Autodesk Inventor part; units mm, degrees
ref_plane "YZ Plane" through (0, 0, 0) normal (1, 0, 0) x (0, 1, 0)
ref_plane "XZ Plane" through (0, 0, 0) normal (0, 1, 0) x (-1, 0, 0)
ref_plane "XY Plane" through (0, 0, 0) normal (0, 0, 1) x (1, 0, 0)
sketch "Sketch1" plane through (0, 0, 0) normal (0, 1, 0) x (-1, 0, 0)
  line L0 (107.2514, 61.1758) -> (-112.4586, 61.1758)
  line L1 (-112.4586, 61.1758) -> (-112.4586, 42.1258)
  line L2 (-112.4586, 42.1258) -> (107.2514, 42.1258)
  line L3 (107.2514, 42.1258) -> (107.2514, 61.1758)
  point P0 (0, 0)
  dimension "d0" = 219.71
  dimension "d1" = 19.05
extrude "Extrusion1" add sketch "Sketch1" along normal blind 139.7
sketch "Sketch2" plane through (-107.2514, 0, 61.1758) normal (0, 0, 1) x (1, 0, 0)
  line L0 (0, 0) -> (219.71, 0)
  line L1 (0, 139.7) -> (219.71, 139.7)
  line L2 (0, 0) -> (0, 139.7)
  line L3 (219.71, 0) -> (219.71, 139.7)
  point P0 (107.2514, 0)
  point P1 (9.525, 76.2)
  point P2 (9.525, 25.4)
  point P3 (210.185, 25.4)
  point P4 (210.185, 76.2)
  dimension "d4" = 0
  dimension "d5" = 0
  dimension "d6" = 0
  dimension "d7" = 0
  dimension "d8" = 25.4
  dimension "d10" = 9.525
  dimension "d11" = 9.525
  dimension "d57" = 50.8
hole "Hole1" at (-97.7264, 76.2, 61.1758) at (-97.7264, 25.4, 61.1758) at (102.9336, 25.4, 61.1758) at (102.9336, 76.2, 61.1758) direction (0, 0, -1) diameter 6.35 end through all
sketch "Sketch3" plane through (-107.2514, 0, 61.1758) normal (0, 0, 1) x (1, 0, 0)
  line L0 (19.05, 133.35) -> (200.66, 133.35)
  line L1 (200.66, 133.35) -> (200.66, 6.35)
  line L2 (200.66, 6.35) -> (19.05, 6.35)
  line L3 (19.05, 6.35) -> (19.05, 133.35)
  line L4 (0, 0) -> (0, 139.7)
  line L5 (219.71, 0) -> (219.71, 139.7)
  line L6 (219.71, 139.7) -> (0, 139.7)
  line L7 (0, 0) -> (219.71, 0)
  point P0 (107.2514, 0)
  dimension "d19" = 19.05
  dimension "d20" = 19.05
  dimension "d21" = 6.35
  dimension "d22" = 6.35
extrude "Extrusion2" cut sketch "Sketch3" against normal blind 6.35 contours L0 L1 L2 L3
sketch "Sketch6" plane through (0, 139.7, 0) normal (0, 1, 0) x (1, 0, 0)
  line L0 (-88.2014, -54.8258) -> (-107.2514, -54.8258)
  line L1 (-107.2514, -54.8258) -> (-107.2514, -42.1258)
  line L2 (-107.2514, -42.1258) -> (-88.2014, -42.1258)
  line L3 (-88.2014, -42.1258) -> (-88.2014, -54.8258)
  line L4 (112.4586, -42.1258) -> (-107.2514, -42.1258)
  line L5 (-107.2514, -42.1258) -> (-107.2514, -61.1758)
  line L6 (112.4586, -54.8258) -> (93.4086, -54.8258)
  line L7 (93.4086, -54.8258) -> (93.4086, -42.1258)
  line L8 (93.4086, -42.1258) -> (112.4586, -42.1258)
  line L9 (112.4586, -42.1258) -> (112.4586, -54.8258)
  line L10 (112.4586, -61.1758) -> (112.4586, -42.1258)
  line L11 (-107.2514, -61.1758) -> (112.4586, -61.1758)
  point P0 (0, 0)
  dimension "d25" = 0
  dimension "d26" = 12.7
  dimension "d27" = 0
  dimension "d28" = 19.05
  dimension "d32" = 19.05
  dimension "d33" = 0
  dimension "d34" = 6.35
extrude "Extrusion3" cut sketch "Sketch6" against normal blind 254 contours L0 L1 L2 L3 | L4 L9 L6 L7
sketch "Sketch7" plane through (0, 0, 0) normal (0, -1, 0) x (1, 0, 0)
  line L0 (112.4586, 61.1758) -> (112.4586, 42.1258)
  line L1 (112.4586, 42.1258) -> (-107.2514, 42.1258)
  line L2 (-107.2514, 42.1258) -> (-107.2514, 61.1758)
  point P0 (0, 0)
  point P1 (61.6586, 51.6508)
  point P2 (-56.4514, 51.6508)
  point P3 (112.4586, 54.8258)
  point P4 (93.4086, 42.1258)
  point P5 (-88.2014, 42.1258)
  point P6 (-107.2514, 54.8258)
  dimension "d37" = 50.8
  dimension "d38" = 9.525
  dimension "d39" = 50.8
  dimension "d40" = 9.525
hole "Hole2" at (61.6586, 0, 51.6508) at (-56.4514, 0, 51.6508) direction (0, 1, 0) diameter 4.9149 depth 25.4 tip angle 118
sketch "Sketch8" plane through (0, 0, 0) normal (0, -1, 0) x (1, 0, 0)
  line L0 (112.4586, 61.1758) -> (112.4586, 42.1258)
  line L1 (112.4586, 42.1258) -> (-107.2514, 42.1258)
  point P0 (0, 0)
  point P1 (-1.8414, 51.6508)
  point P2 (-1.8414, 51.6508)
  point P3 (112.4586, 54.8258)
  point P4 (93.4086, 42.1258)
  point P5 (-88.2014, 42.1258)
  dimension "d48" = 114.3
  dimension "d49" = 9.525
hole "Hole3" at (-1.8414, 0, 51.6508) direction (0, 1, 0) diameter 4.9149 depth 25.4 tip angle 118
sketch "Sketch9" plane through (-107.2514, 0, 61.1758) normal (0, 0, 1) x (1, 0, 0)
  circle A0 centre (210.185, 76.2) radius 3.175
  line L0 (219.71, 0) -> (219.71, 139.7)
  line L1 (0, 0) -> (0, 139.7)
  point P0 (107.2514, 0)
  point P1 (9.525, 127)
  point P2 (210.185, 127)
  dimension "d58" = 0
  dimension "d59" = 50.8
  dimension "d60" = 9.525
  dimension "d61" = 9.525
hole "Hole4" at (-97.7264, 127, 61.1758) at (102.9336, 127, 61.1758) direction (0, 0, -1) diameter 6.35 depth 25.4 tip angle 118
properties part number "TallFrontWall"
Geometry: final body of the model. Coordinates: model frame, mm. A direction names the side the tool comes from. Round coordinates to 2 decimals unless told otherwise and drop trailing zeros. Order: outer loops, then holes, each group sorted by start corner. A loop starts at its lowest first (then second) coordinate and runs counter-clockwise, first axis right, second up. Notation, with made-up numbers: (67, -1.75) - (95, -1.75) arc R21 cw to (95, 21.25) - close; hole circle Ø3 at (86, -7.5). An arc over 180 degrees is marked (long way). Use CSV: the item, a comma, the result in double quotes. Start each with the question number.
Q1. Material intervals for line 1 along X through (y, z) = (127, 59); line 2 along Y through (x, z) = (57, 58.25); line 3 along X through (y, z) = (102, 59.75), sorted ascending. Write a range as from..to.
Q2. Section query C-C (x = 38). Return loops of the section in (y, z), and give its area (3 significant figures).
Q3. Mould query, pull axis X, two halves, no side actions, for faces 1 (the face through (4, 69, 42.126)), 2 (the face through (4, 6.35, 58)), 3 (the face through (112.459, 69, 58)). Classes: +X half, -X half, draft (parallel to the pull), parting line (faces both ways), or undercut.
Q4. First-contact query: pin 1 (9.5 mm diameter, centred on x = 99.5, y = 39, fed in from -Z); pin 2 (4 mm diameter, centred on y = 109, z = 50, fed in from -X); pin 3 (5 mm diameter, centred on x = 102.93, y = 76.2, fed in from +Z); pin 4 (8 mm diameter, centred on x = 77.5, y = 38.5, fed in from +Z). Flat tips, straight axial feed; report the tip coordinate or a pass-through.
Q5. Access query for faces 4 (the face through (1, 133.35, 58)), 5 (the face through (62.6, 12.88, 49.38)), 6 (the face through (93.409, 71, 49)), 7 (the face through (-98, 71, 54.826)). Directions: +Z, -Z, +X, -X, +Y, -Y. A direction counts if a zero-diameter tool reaches every point of the face in a straight line with its end or side. Return the directions, or none.
Result set:
1,line 1,"x = -107.25..-100.9, -94.55..-88.2, 93.41..99.76, 106.11..112.46"
1,line 2,"y = 0..6.35, 133.35..139.7"
1,line 3,"x = -107.25..-88.2, 93.41..112.46"
2,outline,"(0, 42.13) - (139.7, 42.13) - (139.7, 61.18) - (133.35, 61.18) - (133.35, 54.83) - (6.35, 54.83) - (6.35, 61.18) - (0, 61.18) - close"
2,area,"1,850 mm2"
3,face 1,"draft"
3,face 2,"undercut"
3,face 3,"+X half"
4,pin 1,"stops at z = 54.83"
4,pin 2,"stops at x = -88.2"
4,pin 3,"passes through"
4,pin 4,"stops at z = 54.83"
5,face 4,"+Z"
5,face 5,"-Y"
5,face 6,"-Z, +X, +Y, -Y"
5,face 7,"-Z, -X, +Y, -Y"
